Check sheet for the modelled part. Datum: model origin and axes. Units: mm. Face numbers are marked on the shaded views. Round coordinates to 2 decimals unless told otherwise and drop trailing zeros. Write each loop counter-clockwise with the first axis right and the second up, starting at its lowest first coordinate (ties: lowest second). Pieces come first, ordered by that corner, then holes.
Item 1: Cross-section at A-A on z = 4.5. Enter the section's corners in (x, y).
Item 2: Release check for a two-part mould opening along Z. For the marked faces 1 and 2 record: +Z half, -Z half, draft (parallel to the pull), parting line (faces both ways), or undercut.
Item 3: Go/stop test with flat-tipped pins: pin 1 Ø1.5 at (y, z) = (-0.5, -11) entering from -X; pin 2 Ø2.5 at (x, y) = (3.5, 2) entering from +Z; pin 3 Ø5 at (x, z) = (37, -13) entering from -Y. Record where each tip stops, or that it passes through.
Item 4: Cross-section at B-B on x = 20. Enter the section's corners in (y, z).
Item 5: Cross-section at D-D on y = -3.25. Count the separate pieces of the cut face and the enclosed holes in it, plus the area to 3 significant figures.
Item 6: Cross-section at C-C on z = -18. Enter the section's corners in (x, y).
Item 7: Material ranges on line 1 (X direction, y = 1, z = 4); line 2 (Z direction, x = 47.5, y = 2); line 3 (X direction, y = 1.75, z = 46), recorded low to high.
from build123d import *

# Parameters (mm, degrees)
BOSS_EXTRUDE1_DEPTH     = 3
BOSS_EXTRUDE2_DEPTH     = 5
CUT_EXTRUDE1_DEPTH      = 3
SKETCH1_R               = 2
CUT_EXTRUDE2_DEPTH      = 4
CUT_EXTRUDE2_DEPTH_BACK = 6
CUT_EXTRUDE4_DEPTH      = 10
FILLET1_R               = 3
FILLET2_R               = 10
CUT_EXTRUDE5_DEPTH      = 10
SKETCH9_W               = 5
SKETCH9_H               = 21.953318806
SKETCH9_W_2             = 21.953318806
SKETCH9_H_2             = 5
CUT_EXTRUDE6_DEPTH      = 10
FILLET3_R               = 2
SKETCH10_R              = 1.05
CUT_EXTRUDE7_DEPTH      = 10
CUT_EXTRUDE7_DEPTH_BACK = 10
SKETCH11_R              = 4
SKETCH11_R_2            = 1.05
BOSS_EXTRUDE3_DEPTH     = 2
SKETCH13_R              = 4
CUT_EXTRUDE9_DEPTH      = 10


with BuildPart() as part:
    # Sketch3 → Boss-Extrude1 (new body)
    with BuildSketch(Plane(origin=(0, 0, 0), x_dir=(1, 0, 0), z_dir=(0, 1, 0))):
        Polygon((-53.74011537, 31.112698372), (-31.112698372, 53.74011537), (31.112698372, 53.74011537), (53.74011537, 31.112698372), (53.74011537, -31.112698372), (31.112698372, -53.74011537), (-31.112698372, -53.74011537), (-53.74011537, -31.112698372), align=None)
    extrude(amount=BOSS_EXTRUDE1_DEPTH)

    # Sketch4 → Boss-Extrude2 (add)
    with BuildSketch(Plane(origin=(0, 0, 0), x_dir=(-1, 0, 0), z_dir=(0, -1, 0))):
        Polygon((53.74011537, -31.112698372), (31.112698372, -53.74011537), (24.395183951, -47.022600949), (47.022600949, -24.395183951), align=None)
        Polygon((31.112698372, 53.74011537), (24.395183951, 47.022600949), (47.022600949, 24.395183951), (53.74011537, 31.112698372), align=None)
        Polygon((-31.112698372, 53.74011537), (-24.395183951, 47.022600949), (-47.022600949, 24.395183951), (-53.74011537, 31.112698372), align=None)
        Polygon((-47.022600949, -24.395183951), (-53.74011537, -31.112698372), (-31.112698372, -53.74011537), (-24.395183951, -47.022600949), align=None)
    extrude(amount=BOSS_EXTRUDE2_DEPTH)

    # Sketch2 → Cut-Extrude1 (cut)
    with BuildSketch(Plane(origin=(0, 0, 0), x_dir=(1, 0, 0), z_dir=(0, 1, 0))):
        Polygon((-35.355339059, 24.748737342), (-24.748737342, 35.355339059), (-14.142135624, 24.748737342), (-24.748737342, 14.142135624), align=None)
        Polygon((14.142135624, 24.748737342), (24.748737342, 14.142135624), (35.355339059, 24.748737342), (24.748737342, 35.355339059), align=None)
        Polygon((-14.142135624, -24.748737342), (-24.748737342, -14.142135624), (-35.355339059, -24.748737342), (-24.748737342, -35.355339059), align=None)
        Polygon((14.142135624, -24.748737342), (24.748737342, -14.142135624), (35.355339059, -24.748737342), (24.748737342, -35.355339059), align=None)
    extrude(amount=CUT_EXTRUDE1_DEPTH, mode=Mode.SUBTRACT)

    # Sketch1 → Cut-Extrude2 (cut, two sides)
    with BuildSketch(Plane(origin=(0, 0, 0), x_dir=(1, 0, 0), z_dir=(0, 1, 0))) as cut_extrude2_sk:
        with Locations((31.466251763, 46.315494168)):
            Circle(SKETCH1_R)
        with Locations((46.315494168, 31.466251763)):
            Circle(SKETCH1_R)
        with Locations((46.315494168, -31.466251763)):
            Circle(SKETCH1_R)
        with Locations((31.466251763, -46.315494168)):
            Circle(SKETCH1_R)
        with Locations((-31.466251763, -46.315494168)):
            Circle(SKETCH1_R)
        with Locations((-46.315494168, -31.466251763)):
            Circle(SKETCH1_R)
        with Locations((-46.315494168, 31.466251763)):
            Circle(SKETCH1_R)
        with Locations((-31.466251763, 46.315494168)):
            Circle(SKETCH1_R)
    extrude(amount=CUT_EXTRUDE2_DEPTH, mode=Mode.SUBTRACT)
    extrude(cut_extrude2_sk.sketch, amount=-CUT_EXTRUDE2_DEPTH_BACK, mode=Mode.SUBTRACT)

    # Sketch5 → Cut-Extrude4 (cut)
    with BuildSketch(Plane(origin=(0, 0, 0), x_dir=(1, 0, 0), z_dir=(0, 1, 0))):
        Polygon((-53.74011537, -31.112698372), (-33.5, -10.872583002), (-33.5, 10.872583002), (-53.74011537, 31.112698372), align=None)
        Polygon((53.74011537, -31.112698372), (33.5, -10.872583002), (33.5, 10.872583002), (53.74011537, 31.112698372), align=None)
        Polygon((-31.112698372, -53.74011537), (31.112698372, -53.74011537), (10.872583002, -33.5), (-10.872583002, -33.5), align=None)
        Polygon((-31.112698372, 53.74011537), (31.112698372, 53.74011537), (10.872583002, 33.5), (-10.872583002, 33.5), align=None)
    extrude(amount=CUT_EXTRUDE4_DEPTH, mode=Mode.SUBTRACT)

    # Fillet1
    fillet1_edges = [part.edges().sort_by_distance(p)[0] for p in [
        (-53.74011537, -1, -31.112698372),
        (-31.112698372, -1, -53.74011537),
        (31.112698372, -1, -53.74011537),
        (53.74011537, -1, -31.112698372),
        (53.74011537, -1, 31.112698372),
        (31.112698372, -1, 53.74011537),
        (-31.112698372, -1, 53.74011537),
        (-53.74011537, -1, 31.112698372),
        (-47.022600949, -2.5, 24.395183951),
        (-24.395183951, -2.5, 47.022600949),
        (-24.395183951, -2.5, -47.022600949),
        (-47.022600949, -2.5, -24.395183951),
        (47.022600949, -2.5, -24.395183951),
        (24.395183951, -2.5, -47.022600949),
        (24.395183951, -2.5, 47.022600949),
        (47.022600949, -2.5, 24.395183951),
    ]]
    fillet(fillet1_edges, radius=FILLET1_R)

    # Fillet2
    fillet2_edges = [part.edges().sort_by_distance(p)[0] for p in [
        (-33.5, 1.5, 10.872583002),
        (-33.5, 1.5, -10.872583002),
        (33.5, 1.5, -10.872583002),
        (33.5, 1.5, 10.872583002),
        (10.872583002, 1.5, 33.5),
        (-10.872583002, 1.5, 33.5),
        (-10.872583002, 1.5, -33.5),
        (10.872583002, 1.5, -33.5),
    ]]
    fillet(fillet2_edges, radius=FILLET2_R)

    # Sketch8 → Cut-Extrude5 (cut)
    with BuildSketch(Plane.XZ):
        Polygon((-26.5, 10.976659403), (-10.976659403, 26.5), (10.976659403, 26.5), (26.5, 10.976659403), (26.5, -10.976659403), (10.976659403, -26.5), (-10.976659403, -26.5), (-26.5, -10.976659403), align=None)
    extrude(amount=-CUT_EXTRUDE5_DEPTH, mode=Mode.SUBTRACT)

    # Sketch9 → Cut-Extrude6 (cut)
    with BuildSketch(Plane.XZ):
        with Locations((-27.5, 0)):
            Rectangle(SKETCH9_W, SKETCH9_H)
        with Locations((0, 27.5)):
            Rectangle(SKETCH9_W_2, SKETCH9_H_2)
        with Locations((27.5, 0)):
            Rectangle(SKETCH9_W, SKETCH9_H)
        with Locations((0, -27.5)):
            Rectangle(SKETCH9_W_2, SKETCH9_H_2)
    extrude(amount=-CUT_EXTRUDE6_DEPTH, mode=Mode.SUBTRACT)

    # Fillet3
    fillet3_edges = [part.edges().sort_by_distance(p)[0] for p in [
        (-26.5, 1.5, -10.976659403),
        (-26.5, 1.5, 10.976659403),
        (-10.976659403, 1.5, 26.5),
        (10.976659403, 1.5, 26.5),
        (26.5, 1.5, 10.976659403),
        (26.5, 1.5, -10.976659403),
        (10.976659403, 1.5, -26.5),
        (-10.976659403, 1.5, -26.5),
        (-30, 1.5, -10.976659403),
        (-30, 1.5, 10.976659403),
        (-10.976659403, 1.5, 30),
        (10.976659403, 1.5, 30),
        (30, 1.5, 10.976659403),
        (30, 1.5, -10.976659403),
        (10.976659403, 1.5, -30),
        (-10.976659403, 1.5, -30),
    ]]
    fillet(fillet3_edges, radius=FILLET3_R)

    # Sketch10 → Cut-Extrude7 (cut, two sides)
    with BuildSketch(Plane(origin=(0, 0, 0), x_dir=(1, 0, 0), z_dir=(0, 1, 0))) as cut_extrude7_sk:
        with Locations((36.239222536, 36.239222536)):
            Circle(SKETCH10_R)
        with Locations((-36.239222536, -36.239222536)):
            Circle(SKETCH10_R)
        with Locations((-36.239222536, 36.239222536)):
            Circle(SKETCH10_R)
        with Locations((36.239222536, -36.239222536)):
            Circle(SKETCH10_R)
    extrude(amount=CUT_EXTRUDE7_DEPTH, mode=Mode.SUBTRACT)
    extrude(cut_extrude7_sk.sketch, amount=-CUT_EXTRUDE7_DEPTH_BACK, mode=Mode.SUBTRACT)

    # Sketch11 → Boss-Extrude3 (add)
    with BuildSketch(Plane.XZ):
        with Locations((36.239222536, -36.239222536)):
            Circle(SKETCH11_R)
        with Locations((36.239222536, -36.239222536)):
            Circle(SKETCH11_R_2, mode=Mode.SUBTRACT)
        with Locations((-36.239222536, 36.239222536)):
            Circle(SKETCH11_R)
        with Locations((-36.239222536, 36.239222536)):
            Circle(SKETCH11_R_2, mode=Mode.SUBTRACT)
        with Locations((-36.239222536, -36.239222536)):
            Circle(SKETCH11_R)
        with Locations((-36.239222536, -36.239222536)):
            Circle(SKETCH11_R_2, mode=Mode.SUBTRACT)
        with Locations((36.239222536, 36.239222536)):
            Circle(SKETCH11_R)
        with Locations((36.239222536, 36.239222536)):
            Circle(SKETCH11_R_2, mode=Mode.SUBTRACT)
    extrude(amount=BOSS_EXTRUDE3_DEPTH)

    # Sketch13 → Cut-Extrude9 (cut)
    with BuildSketch(Plane.XZ.offset(2)):
        with Locations((-36.239222536, 36.239222536)):
            Circle(SKETCH13_R)
        with Locations((36.239222536, 36.239222536)):
            Circle(SKETCH13_R)
        with Locations((36.239222536, -36.239222536)):
            Circle(SKETCH13_R)
        with Locations((-36.239222536, -36.239222536)):
            Circle(SKETCH13_R)
    extrude(amount=CUT_EXTRUDE9_DEPTH, mode=Mode.SUBTRACT)


solid = part.part
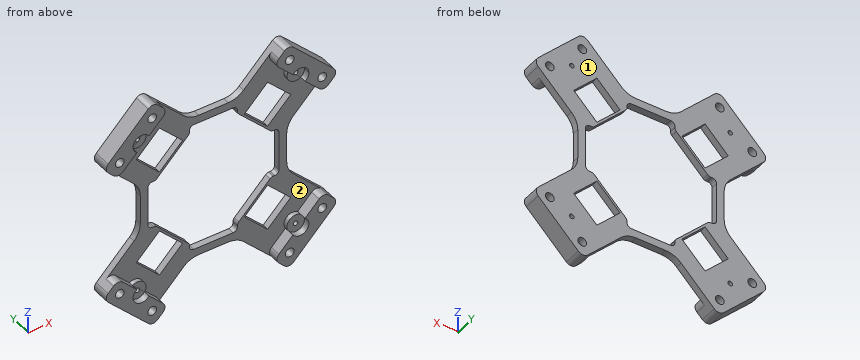
Response values:
1. outline: (-33.5, 0) - (-30, 0) - (-30, 3) - (-33.5, 3) - close; (30, 0) - (33.5, 0) - (33.5, 3) - (30, 3) - close
2. face 1: draft
2. face 2: undercut
3. pin 1: stops at x = -34.74
3. pin 2: stops at z = 33.5
3. pin 3: stops at y = 0
4. outline: (0, -42.63) - (3, -42.63) - (3, -30.61) - (0, -30.61) - close; (0, -18.89) - (3, -18.89) - (3, -17.48) - (0, -17.48) - close; (0, 17.48) - (3, 17.48) - (3, 18.89) - (0, 18.89) - close; (0, 30.61) - (3, 30.61) - (3, 42.63) - (0, 42.63) - close
5. separate pieces: 4
5. enclosed holes: 8
5. area: 960 mm2
6. outline: (-40.63, 0) - (-28.61, 0) - (-28.61, 3) - (-40.63, 3) - close; (-20.89, 0) - (-19.48, 0) - (-19.48, 3) - (-20.89, 3) - close; (19.48, 0) - (20.89, 0) - (20.89, 3) - (19.48, 3) - close; (28.61, 0) - (40.63, 0) - (40.63, 3) - (28.61, 3) - close
7. line 1: x = -33.5 to -30, 30 to 33.5
7. line 2: z = -37.35 to -33.08, -29.85 to -24.87, 24.87 to 29.85, 33.08 to 37.35
7. line 3: x = -38.85 to -33.44, -29.49 to -23.37, 23.37 to 29.49, 33.44 to 38.85
